```python
from build123d import *

# Parameters (mm, degrees)
CONECUT_DEPTH      = 28.836502766
CONECUT_DEPTH_BACK = 28.836502766


with BuildPart() as part:
    # BaseBody: sweep along a path in PathSke
    with BuildLine(Plane.XY) as basebody_path:
        Line((23.665, 1.45), (3.665, 1.45))
        ThreePointArc((3.665, 1.45), (2.628048973, 1.626517109), (1.707905138, 2.136184692))
        ThreePointArc((1.707905138, 2.136184692), (-2.735, 0), (1.707905138, -2.136184692))
        ThreePointArc((1.707905138, -2.136184692), (2.628048973, -1.626517109), (3.665, -1.45))
        Line((3.665, -1.45), (27.665, -1.45))
    # SectionSke → BaseBody (sweep)
    with BuildSketch(Plane(origin=(23.665, 1.45, 0), x_dir=(0, 0, -1), z_dir=(1, 0, 0))):
        with BuildLine():
            Line((-1.197737868, -1.448), (1.197737868, -1.448))
            ThreePointArc((1.197737868, -1.448), (1.375163447, -1.364356291), (1.423540908, -1.174262295))
            ThreePointArc((1.423540908, -1.174262295), (0, 0), (-1.423540908, -1.174262295))
            ThreePointArc((-1.423540908, -1.174262295), (-1.375163447, -1.364356291), (-1.197737868, -1.448))
        make_face()
    sweep(path=basebody_path.line)

    # ConeCutSke → ConeCut (cut, two sides: drawn at the far end of the back side and taken through both)
    with BuildSketch(Plane.XY.offset(-CONECUT_DEPTH_BACK)):
        Polygon((22.633898934, 1.46), (27.675, 1.46), (27.675, -1.46), (26.633898934, -1.46), (27.665, -0.862868852), (26.633898934, 0), (22.633898934, 0), (23.665, 0.862868852), align=None)
    extrude(amount=CONECUT_DEPTH + CONECUT_DEPTH_BACK, mode=Mode.SUBTRACT)


solid = part.part
```
Geometry check sheet. Reference: the model listing, model coordinates, mm. Coordinates: 2 decimals unless noted, no trailing zeros. Write each loop counter-clockwise with the first axis right and the second up, starting at its lowest first coordinate (ties: lowest second). Pieces come first, ordered by that corner, then holes. Notation, with made-up numbers: M -29.75,70.25 L -3.75,70.25 A22 cw -3.75,78.25 Z; hole C 81,22.25 d11. An arc over 180 degrees is marked long. Use one line per item in the form item = value. Start each with the question number.
1) Section check B-B on x = 25. Enter the section's corners in (y, z).
2) Thickness scan on probe 1 along Y at (x, z) = (0, 0.1); probe 2 along Y at (x, z) = (0, 0.6); probe 3 along Z at (x, y) = (1, 2.1). Record the ranges inside material, lowest first. Write a range as from..to.
3) Go/stop test with a flat-tipped pin: pin 1 Ø0.7 at (x, z) = (12, 0) entering from -Y. Record where the tip stops, or that it passes through.
4) Release check for a two-part mould opening along Y. For faces 1 (the cylindrical face through (15.83, -1.45, 0.03)), 2 (the cylindrical face through (2.169, 0.253, -0.017)), 3 (the cylindrical face through (13.52, 1.45, 0.03)) record: pulls with the +Y half, pulls with the -Y half, needs draft (parallel to the pull), parting line crosses it, or undercut.
5) Section check A-A on x = 21.5. Enter the section's corners in (y, z), and give its area (3 significant figures).
Responses:
q1.outline = M -0.28,-1.42 A0.23 ccw 0,-1.2 L 0,1.2 A0.23 ccw -0.28,1.42 A1.45 ccw Z
q2.probe_1 = -2.73..-1.29, 1.29..2.73
q2.probe_2 = -2.61..-1.29, 1.29..2.61
q2.probe_3 = -1.01..1.01
q3.pin_1 = -1.45
q4.face_1 = pulls with the -Y half
q4.face_2 = undercut
q4.face_3 = pulls with the +Y half
q5.outline = M -0.28,-1.42 A0.23 ccw 0,-1.2 L 0,1.2 A0.23 ccw -0.28,1.42 A1.45 ccw Z; M 0,-1.2 A0.23 ccw 0.28,-1.42 A1.45 ccw 0.28,1.42 A0.23 ccw 0,1.2 Z
q5.area = 6.53 mm2
